Verification items for the finished model (mm, model axes). A direction names the side the tool comes from. Round coordinates to 2 decimals unless told otherwise and drop trailing zeros. Write each loop counter-clockwise with the first axis right and the second up, starting at its lowest first coordinate (ties: lowest second). Pieces come first, ordered by that corner, then holes.
from build123d import *

# Parameters (mm, degrees)
BOX043_W               = 30
BOX043_H               = 64
BOX043_DEPTH           = 102
BOX042_W               = 175
BOX042_H               = 120
BOX042_DEPTH           = 23
CUT013_ROLL_ANGLE      = -90
CUT013_PLACEMENT_ANGLE = -180


with BuildPart() as cube038:
    # Box043 → Box043 (new body)
    with BuildSketch(Plane(origin=(28, 18, 27), x_dir=(0, 0, -1), z_dir=(1, 0, 0))):
        with Locations((15, 32)):
            Rectangle(BOX043_W, BOX043_H)
    extrude(amount=BOX043_DEPTH)


with BuildPart() as obj1:
    # Box042 → Box042 (new body)
    with BuildSketch(Plane.XY):
        with Locations((87.5, 60)):
            Rectangle(BOX042_W, BOX042_H)
    extrude(amount=BOX042_DEPTH)

    # Cut013: cut Cube038
    add(cube038.part, mode=Mode.SUBTRACT)


with BuildPart() as obj1_1:
    # Cut013 roll: moved
    add(obj1.part.rotate(Axis((0, 0, 0), (1, 0, 0)), CUT013_ROLL_ANGLE))


with BuildPart() as obj1_2:
    # Cut013 placement: moved
    add(obj1_1.part.moved(Location((185, 241, 13))).rotate(Axis((185, 241, 13), (0, 0, 1)), CUT013_PLACEMENT_ANGLE))


solid = obj1_2.part
Q1. Tool access check on faces 4 (the flat face through (185, 230, -46)), 5 (the flat face through (107, 229, -5)). Record the directions out of +Z, -Z, +X, -X, +Y, -Y that give a thin tool (end or side, any length) a straight path to the whole face; none if there is none.
Recorded:
face 4: +Z, -Z, +X, +Y, -Y
face 5: +Y, -Y
Q2. Material ranges on line 1 along X through (y, z) = (220, -45); line 2 along Z through (x, y) = (128.5, 239.25), recorded low to high.
Recorded:
line 1: x = 10 to 55, 157 to 185
line 2: z = -107 to -69, -5 to 13
Q3. Sectioned sample at B-B (x = 75). Enter the section's corners in (y, z).
Recorded:
outline: (218, -107) - (241, -107) - (241, -69) - (218, -69) - close; (218, -5) - (241, -5) - (241, 13) - (218, 13) - close
Q4. Release check for a two-part mould opening along X. For faces 1 (the flat face through (10, 230, -46)), 2 (the flat face through (107, 229, -69)), 3 (the flat face through (99, 230, 13)) record: released by +X, released by -X, zero draft, split by the parting line, or undercut.
Recorded:
face 1: released by -X
face 2: undercut
face 3: zero draft
Q5. Sectioned sample at A-A (z = -31.5). Enter the section's corners in (x, y).
Recorded:
outline: (10, 218) - (55, 218) - (55, 241) - (10, 241) - close; (157, 218) - (185, 218) - (185, 241) - (157, 241) - close
Q6. Sectioned sample at C-C (y = 238). Enter the section's corners in (x, z), plus the area to 3 significant figures.
Recorded:
outline: (10, -107) - (185, -107) - (185, 13) - (10, 13) - close; hole (55, -69) - (157, -69) - (157, -5) - (55, -5) - close
area: 14,500 mm2
